```python
from build123d import *

# Parameters (mm, degrees)
F0_R     = 32.5
F1_DEPTH = 150
F2_R     = 42.5
F2_R_2   = 32.5
F3_DEPTH = 650
F4_R     = 32.5
F5_DEPTH = 150


with BuildPart() as f1:
    # F0 (on Front) → F1 (new body)
    with BuildSketch(Plane.XZ):
        Circle(F0_R)
    extrude(amount=F1_DEPTH)

    # F2 (on face) → F3 (join)
    with BuildSketch(Plane.XZ.offset(150)):
        Circle(F2_R)
        Circle(F2_R_2, mode=Mode.SUBTRACT)
        Circle(F2_R_2)
    extrude(amount=F3_DEPTH)

    # F4 (on face) → F5 (join)
    with BuildSketch(Plane.XZ.offset(800)):
        Circle(F4_R)
    extrude(amount=F5_DEPTH)


solid = f1.part
```
Part model, mm, in its own coordinate system. A direction names the side the tool comes from. Coordinates: 2 decimals unless noted, no trailing zeros. Order: outer loops, then holes, each group sorted by start corner. A loop starts at its lowest first (then second) coordinate and runs counter-clockwise, first axis right, second up. Notation, with made-up numbers: (9, -12) - (41, -12) arc R23 ccw to (41, -2) - close; hole circle Ø1 at (67.25, -8). An arc over 180 degrees is marked (long way). Return JSON: item names as keys, results as strings. Group by question number.
Item 1: Which spindle directions (+Z, -Z, +X, -X, +Y, -Y) get a long thin tool onto all of the face, cutting with end or side? Do faces 1 (the face through (31, -873.95, 9.76)), 2 (the face through (-9.6, -150, -31.3)), 3 (the face through (0, 0, 0)). Say none if no direction does.
Item 2: Cut at A-A (z = 0). List the corners of the cut face in (x, y).
Item 3: Drill centre lines: probe 1 along Y at (x, z) = (23, 29); probe 2 along Z at (x, y) = (27.5, -341.5); probe 3 along X at (y, z) = (-681, 3). Where is each one in solid material? Low to high. Write a range as from..to.
Item 4: Cut at C-C (y = -607). List the corners of the cut face in (x, z), plus the area to 3 significant figures.
Item 5: Cut at D-D (y = -841). List the corners of the cut face in (x, z).
Item 6: Pin check, flat tips, straight feed: pin 1 (8 mm diameter, centred on x = 4, y = -424.5, fed in from +Z); pin 2 (1 mm diameter, centred on y = -553.5, z = -12.5, fed in from -X); pin 3 (4 mm diameter, centred on y = -113, z = 16.5, fed in from +X). Stop position of each tip, or through.
Item 7: Cut at B-B (x = 0). List the corners of the cut face in (y, z), plus the area to 4 significant figures.
Check values:
{
 "1": {"face 1": "-Y", "face 2": "+Y", "face 3": "+Z, -Z, +X, -X, +Y"},
 "2": {"outline": "(-42.5, -800) - (-32.5, -800) - (-32.5, -950) - (32.5, -950) - (32.5, -800) - (42.5, -800) - (42.5, -150) - (32.5, -150) - (32.5, 0) - (-32.5, 0) - (-32.5, -150) - (-42.5, -150) - close"},
 "3": {"probe 1": "y = -800..-150", "probe 2": "z = -32.4..32.4", "probe 3": "x = -42.39..42.39"},
 "4": {"outline": "circle Ø85 at (0, 0)", "area": "5,670 mm2"},
 "5": {"outline": "circle Ø65 at (0, 0)"},
 "6": {"pin 1": "stops at z = 42.5", "pin 2": "stops at x = -40.77", "pin 3": "stops at x = 29.09"},
 "7": {"outline": "(-950, -32.5) - (-800, -32.5) - (-800, -42.5) - (-150, -42.5) - (-150, -32.5) - (0, -32.5) - (0, 32.5) - (-150, 32.5) - (-150, 42.5) - (-800, 42.5) - (-800, 32.5) - (-950, 32.5) - close", "area": "74,750 mm2"}
}
